Here's the drawing with two shaded views (mm, measured from the low corner). I have some questions. A direction names the side the tool comes from. Round coordinates to 2 decimals unless told otherwise and drop trailing zeros. Write each loop counter-clockwise with the first axis right and the second up, starting at its lowest first coordinate (ties: lowest second). Pieces come first, ordered by that corner, then holes. Notation, with made-up numbers: (-1.5, 34.5) -> (40.5, 34.5) arc R19 ccw to (40.5, 63.5) -> close; hole circle Ø3 at (3.5, 69.25). An arc over 180 degrees is marked (long way). Use CSV: the item, a comma, the result in double quotes.
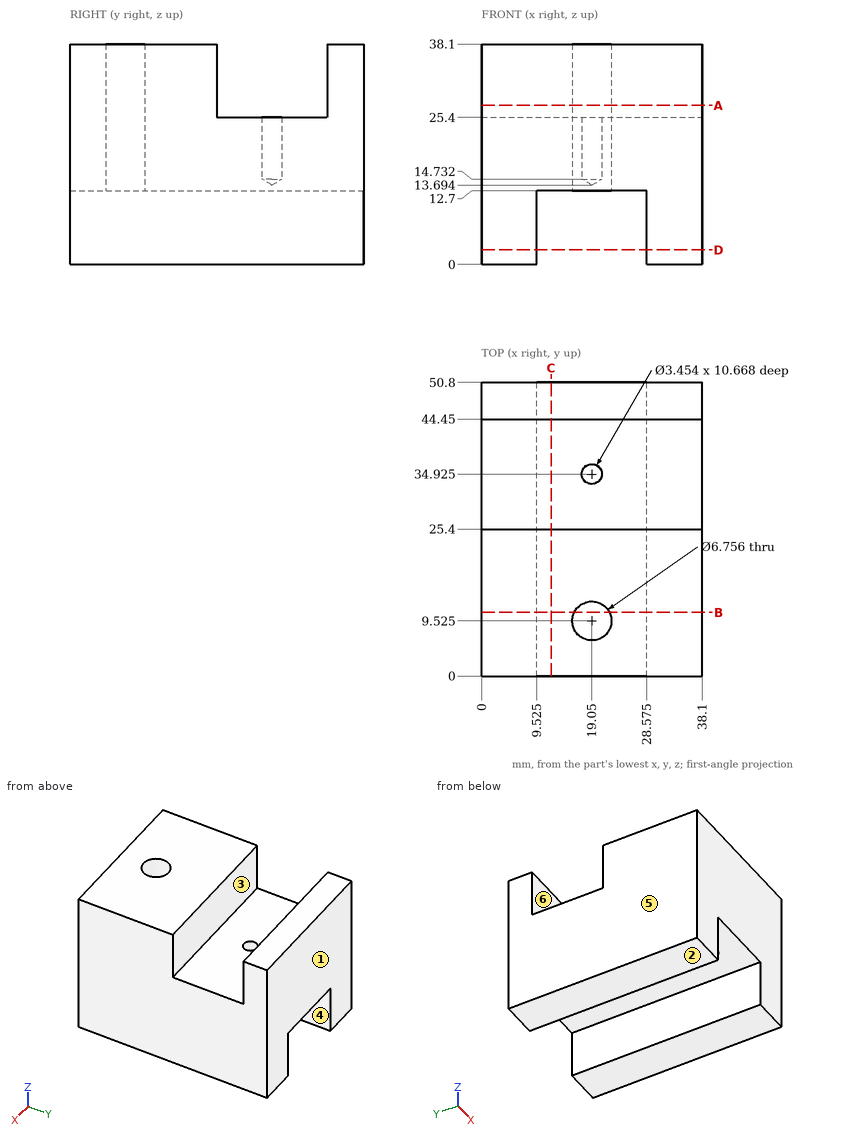
Q1. Suppose I cut it at C-C (x = 12). Write out the boundary of the cut face in (y, z).
Resolved:
outline,"(0, 12.7) -> (50.8, 12.7) -> (50.8, 38.1) -> (44.45, 38.1) -> (44.45, 25.4) -> (25.4, 25.4) -> (25.4, 38.1) -> (0, 38.1) -> close"
Q2. Suppose I cut it at A-A (z = 27.5). Count the separate pieces of the cut face and the enclosed holes in it, and give its area (3 significant figures).
Resolved:
separate pieces,"2"
enclosed holes,"1"
area,"1,170 mm^2"
Q3. Will these pins go through, and if not, where does the flat tip stop? P1, Ø5.5, axis at x = 19.05, y = 9.525, coming from the +Z side; P2, Ø10, axis at x = 20, y = 32, coming from the -Z side; P3, Ø15, axis at x = 20.5, y = 35, coming from the +Z side; P4, Ø2, axis at x = 19.05, y = 34.925, coming from the +Z side (1 decimal).
Resolved:
P1,"passes through"
P2,"stops at z = 12.7"
P3,"stops at z = 25.4"
P4,"stops at z = 14.3"
Q4. Suppose I cut it at B-B (y = 11). Write out the boundary of the cut face in (x, z) (1 decimal), and give its area (3 significant figures).
Resolved:
outline,"(0, 0) -> (9.5, 0) -> (9.5, 12.7) -> (16, 12.7) -> (16, 38.1) -> (0, 38.1) -> close; (22.1, 12.7) -> (28.6, 12.7) -> (28.6, 0) -> (38.1, 0) -> (38.1, 38.1) -> (22.1, 38.1) -> close"
area,"1,060 mm^2"
Q5. Please list where these lines run through material, in increasing order: probe 1 along Y at (x, z) = (19, 25); probe 2 along Y at (x, z) = (19, 28); probe 3 along Y at (x, z) = (32.5, 35).
Resolved:
probe 1,"y = 0 to 6.15, 12.9 to 33.2, 36.65 to 50.8"
probe 2,"y = 0 to 6.15, 12.9 to 25.4, 44.45 to 50.8"
probe 3,"y = 0 to 25.4, 44.45 to 50.8"
Q6. If we mould it in two halves opening along Y, with no side actions, what happens to the marked faces 1, 2 and 3? For each: released by +Y, released by -Y, zero draft, split by the parting line, or undercut.
Resolved:
face 1,"released by +Y"
face 2,"zero draft"
face 3,"undercut"
Q7. On a 3-axis mill with a long thin cutter (end or side, diameter ignored), from which of +Z, -Z, +X, -X, +Y, -Y can I reach the whole of each face in a straight line? I mean the marked faces 4, 5 and 6. Say none if no direction works.
Resolved:
face 4,"-Z, +Y, -Y"
face 5,"+Z, -Z, -X, +Y, -Y"
face 6,"+Z, +X, -X"
Q8. Suppose I cut it at D-D (z = 2.5). Write out the boundary of the cut face in (x, y) (1 decimal).
Resolved:
outline,"(0, 0) -> (9.5, 0) -> (9.5, 50.8) -> (0, 50.8) -> close; (28.6, 0) -> (38.1, 0) -> (38.1, 50.8) -> (28.6, 50.8) -> close"
